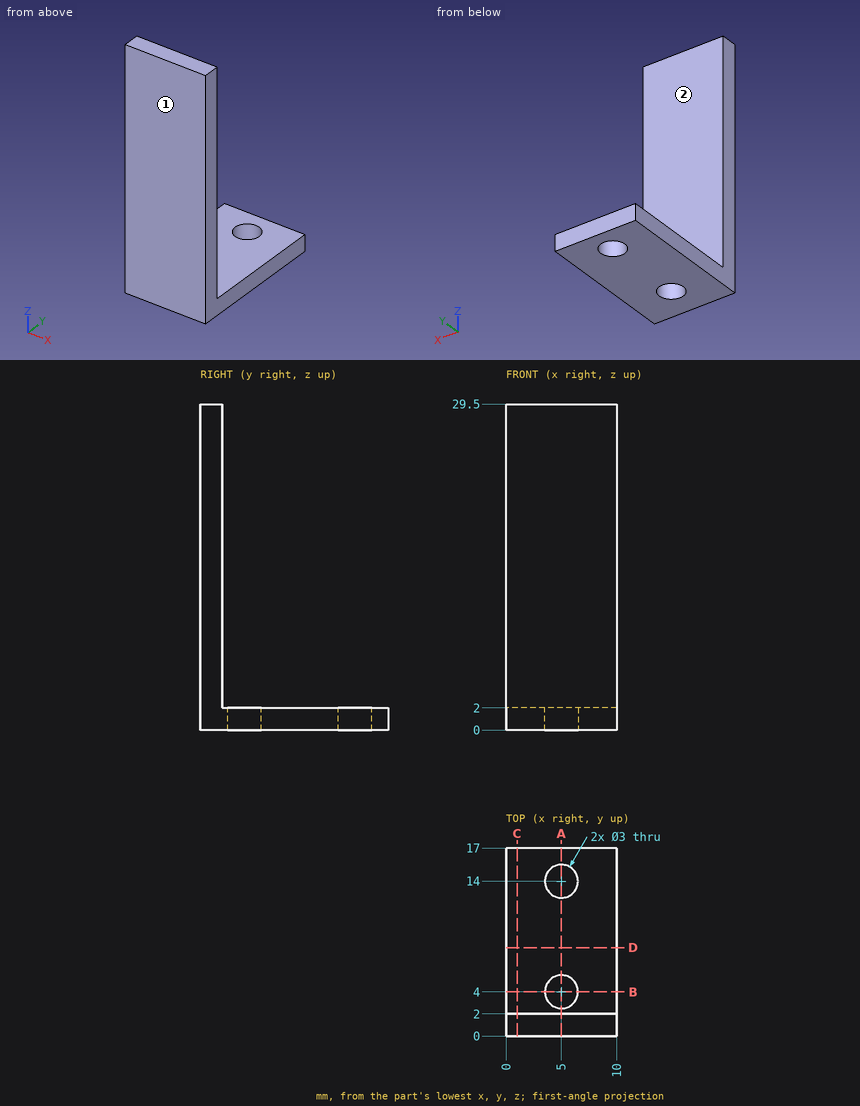
Verification items for this drawing (mm, ordinates from the low corner). A direction names the side the tool comes from. Give positions to 0.01 mm unless a question says otherwise; leave off trailing zeros. Loops run counter-clockwise (first coordinate to the right, second up) from the corner with the lowest first, then second, coordinate; pieces in that order, holes last. Notation, with made-up numbers: (86, 70) - (110, 70) arc R21 cw to (110, 103) - close; hole circle Ø5 at (65.5, 83). An arc over 180 degrees is marked (long way). Write item = value, one per line. Start each with the question number.
Q1. Cross-section at D-D, the plane y = 8. Enter the section's corners in (x, z).
Q2. Thickness scan on line 1 (Y direction, x = 5, z = 0.95); line 2 (Y direction, x = 7.75, z = 4.75). Record the ranges inside material, lowest first.
Q3. Cross-section at B-B, the plane y = 4. Enter the section's corners in (x, z).
Q4. Depth check by flat-ended pin: P1, Ø4, axis at x = 7, z = 17.5, coming from the -Y side; P2, Ø3.5, axis at x = 5, y = 14, coming from the +Z side; P3, Ø1, axis at y = 14.5, z = 4, coming from the +X side; P4, Ø3, axis at x = 6.5, z = 17.5, coming from the +Y side. Enter the tip coordinate at first touch or a pass-through.
Q5. Tool access check on the marked faces 1 and 2. Record the directions out of +Z, -Z, +X, -X, +Y, -Y that give a thin tool (end or side, any length) a straight path to the whole face; none if there is none.
Q6. Cross-section at C-C, the plane x = 1. Enter the section's corners in (y, z).
Q7. Cross-section at A-A, the plane x = 5. Enter the section's corners in (y, z).
Answer key:
q1.outline = (0, 0) - (10, 0) - (10, 2) - (0, 2) - close
q2.line_1 = 0 to 2.5, 5.5 to 12.5, 15.5 to 17
q2.line_2 = 0 to 2
q3.outline = (0, 0) - (3.5, 0) - (3.5, 2) - (0, 2) - close; (6.5, 0) - (10, 0) - (10, 2) - (6.5, 2) - close
q4.P1 = 0
q4.P2 = 2
q4.P3 = through
q4.P4 = 2
q5.face_1 = +Z, -Z, +X, -X, -Y
q5.face_2 = +Z, +X, -X, +Y
q6.outline = (0, 0) - (17, 0) - (17, 2) - (2, 2) - (2, 29.5) - (0, 29.5) - close
q7.outline = (0, 0) - (2.5, 0) - (2.5, 2) - (2, 2) - (2, 29.5) - (0, 29.5) - close; (5.5, 0) - (12.5, 0) - (12.5, 2) - (5.5, 2) - close; (15.5, 0) - (17, 0) - (17, 2) - (15.5, 2) - close
